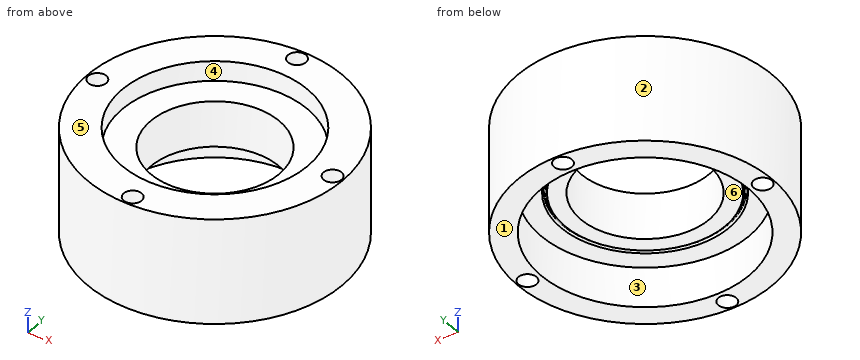
from build123d import *

# Parameters (mm, degrees)
F2_R     = 4.5
F3_DEPTH = 53


with BuildPart() as f1:
    # F0 (on Front) → F1 (revolve)
    with BuildSketch(Plane.XZ):
        with BuildLine():
            Line((52.25, 0), (64, 0))
            Line((64, 0), (64, 53))
            Line((64, 53), (46.5, 53))
            Line((46.5, 53), (46.5, 43))
            Line((46.5, 43), (32.25, 43))
            Line((32.25, 43), (32.25, 20))
            Line((32.25, 20), (40.25, 20))
            Line((40.25, 20), (40.91718, 21.00077))
            ThreePointArc((40.91718, 21.00077), (41.25, 21.17889), (41.58282, 21.00077))
            Line((41.58282, 21.00077), (42.25, 20))
            Line((42.25, 20), (52.25, 20))
            Line((52.25, 20), (52.25, 0))
        make_face()
    revolve(axis=Axis((0, 0, 26.5), (0, 0, 1)))

    # F2 (on face) → F3 (cut)
    with BuildSketch(Plane.XY.offset(53)):
        with Locations((0, 58.8)):
            Circle(F2_R)
        with Locations((58.8, 0)):
            Circle(F2_R)
        with Locations((0, -58.899999)):
            Circle(F2_R)
        with Locations((-58.8, 0)):
            Circle(F2_R)
    extrude(amount=-F3_DEPTH, mode=Mode.SUBTRACT)


solid = f1.part
Design review of the part built by this model. Coordinates are the model's own, in mm. Face numbers are marked on the shaded views. A direction names the side the tool comes from. Coordinates: 2 decimals unless noted, no trailing zeros. Loops run counter-clockwise (first coordinate to the right, second up) from the corner with the lowest first, then second, coordinate; pieces in that order, holes last.
Item 1: Wall thickness on L1, parallel to Y at x = 0, z = 18.5; L2, parallel to X at y = -3, z = 30.5; L3, parallel to Z at x = 22, y = 24.5: over which ranges is each line inside the solid? List them lowest first.
Completed:
L1: y = -64 to -63.4, -54.4 to -52.25, 52.25 to 54.3, 63.3 to 64
L2: x = -63.93 to -62.15, -55.45 to -32.11, 32.11 to 55.45, 62.15 to 63.93
L3: z = 20 to 43
Item 2: Add section C-C (y = -58.9). Write out the cut boundary in (x, z).
Completed:
outline: (-25.04, 0) - (-4.5, 0) - (-4.5, 53) - (-25.04, 53) - close; (4.5, 0) - (25.04, 0) - (25.04, 53) - (4.5, 53) - close
Item 3: Draft analysis for pull direction Y (two halves, no side actions). For the marked faces 1, 2 and 3, state which applies: pulls with the +Y half, pulls with the -Y half, needs draft (parallel to the pull), parting line crosses it, or undercut.
Completed:
face 1: needs draft
face 2: parting line crosses it
face 3: undercut
Item 4: For the marked faces 4, 5 and 6, list the 3-axis set-ups (+Z, -Z, +X, -X, +Y, -Y) from which the entire face can be reached by the end or side of a thin tool; tool diameter is ignored.
Completed:
face 4: +Z
face 5: +Z, +X, -X, +Y, -Y
face 6: -Z
Item 5: Add section A-A (y = 0). Give the number of separate pieces and of enclosed holes in the cut face, and give its area (3 significant figures).
Completed:
separate pieces: 4
enclosed holes: 0
area: 1,320 mm2
Item 6: Clearance check with flat-ended pins moving along their axes: pin 1 (7 mm diameter, centred on x = 0, y = 58.8, fed in from -Z); pin 2 (14.5 mm diameter, centred on x = 0, y = -58.9, fed in from -Z); pin 3 (5 mm diameter, centred on x = 40.5, z = 16.5, fed in from +Y); pin 4 (6 mm diameter, centred on x = 0.5, z = 8, fed in from -Y). State where each tip first meets the part, or that it passes through.
Completed:
pin 1: passes through
pin 2: stops at z = 0
pin 3: stops at y = 51.5
pin 4: stops at y = -64
Item 7: Add section D-D (z = 6.5). Write out the cut boundary in (x, y).
Completed:
outline: circle Ø128 at (0, 0); hole circle Ø9 at (-58.8, 0); hole circle Ø104.5 at (0, 0); hole circle Ø9 at (0, -58.9); hole circle Ø9 at (0, 58.8); hole circle Ø9 at (58.8, 0)
